The listing builds one solid part. Answer for the finished solid, in the listing's coordinates (mm). Coordinates: 2 decimals unless noted, no trailing zeros. Loops run counter-clockwise (first coordinate to the right, second up) from the corner with the lowest first, then second, coordinate; pieces in that order, holes last. Notation, with made-up numbers: (15.25, 14.5) - (53.25, 14.5) arc R29 ccw to (53.25, 48.5) - close; hole circle Ø7 at (88, 24.25). An arc over 180 degrees is marked (long way). Write each question's results on one line, items separated by ' | '. Start each with the question number.
(1) Find section C-C on z = 14.25. Determine the outline of the cut face in (x, y).
(2) Find section B-B on x = -57.5. Determine the outline of the cut face in (y, z).
(3) Given pin 1 Ø5.5 at (x, y) = (-57.5, 60) entering from +Z; pin 2 Ø12.5 at (x, y) = (57.5, -60) entering from -Z; pin 3 Ø5.5 at (x, y) = (-58.5, -59) entering from +Z, each flat-ended and moving along its own axis, determine where each tip first touches the part or whether it passes through.
(4) Consider line 1 (Y direction, x = 57.5, z = 13.25); line 2 (Y direction, x = -57.5, z = 5.75); line 3 (X direction, y = -62.5, z = 7). Determine where each line is inside the solid, lowest interval first. Write a range as from..to.
(5) Find section A-A on y = -60. Determine the outline of the cut face in (x, z).
from build123d import *

# Parameters (mm, degrees)
SKETCH1_W                                           = 130
SKETCH1_H                                           = 150
EXTRUDE1_DEPTH                                      = 16
CBORE_FOR_M6_HEX_SOCKET_HEAD_CAP_SCREW1_D           = 6.6
CBORE_FOR_M6_HEX_SOCKET_HEAD_CAP_SCREW1_CBORE_D     = 11
CBORE_FOR_M6_HEX_SOCKET_HEAD_CAP_SCREW1_CBORE_DEPTH = 6.4


with BuildPart() as part:
    # Sketch1 → Extrude1 (new body)
    with BuildSketch(Plane.XY):
        Rectangle(SKETCH1_W, SKETCH1_H)
    extrude(amount=EXTRUDE1_DEPTH)

    # CBORE for M6 Hex Socket Head Cap Screw1 (through all)
    with Locations(Plane.XY.offset(16)):
        with Locations((-57.5, 60), (-57.5, 0), (-57.5, -60), (57.5, -60), (57.5, 0), (57.5, 60)):
            CounterBoreHole(CBORE_FOR_M6_HEX_SOCKET_HEAD_CAP_SCREW1_D / 2, CBORE_FOR_M6_HEX_SOCKET_HEAD_CAP_SCREW1_CBORE_D / 2, CBORE_FOR_M6_HEX_SOCKET_HEAD_CAP_SCREW1_CBORE_DEPTH)


solid = part.part
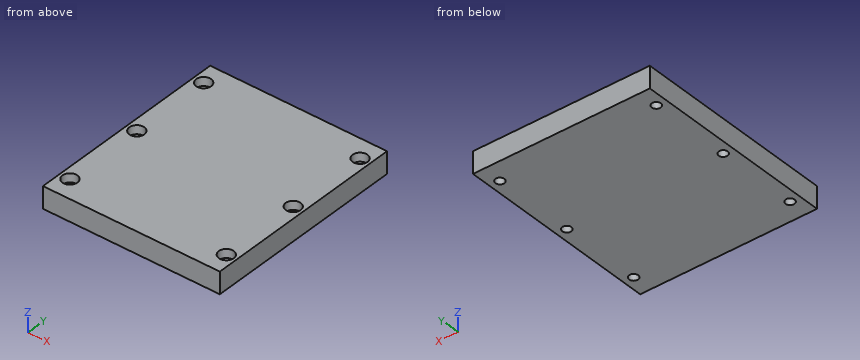
Values:
1) outline: (-65, -75) - (65, -75) - (65, 75) - (-65, 75) - close; hole circle Ø11 at (-57.5, -60); hole circle Ø11 at (-57.5, 0); hole circle Ø11 at (-57.5, 60); hole circle Ø11 at (57.5, -60); hole circle Ø11 at (57.5, 0); hole circle Ø11 at (57.5, 60)
2) outline: (-75, 0) - (-63.3, 0) - (-63.3, 9.6) - (-65.5, 9.6) - (-65.5, 16) - (-75, 16) - close; (-56.7, 0) - (-3.3, 0) - (-3.3, 9.6) - (-5.5, 9.6) - (-5.5, 16) - (-54.5, 16) - (-54.5, 9.6) - (-56.7, 9.6) - close; (3.3, 0) - (56.7, 0) - (56.7, 9.6) - (54.5, 9.6) - (54.5, 16) - (5.5, 16) - (5.5, 9.6) - (3.3, 9.6) - close; (63.3, 0) - (75, 0) - (75, 16) - (65.5, 16) - (65.5, 9.6) - (63.3, 9.6) - close
3) pin 1: passes through | pin 2: stops at z = 0 | pin 3: stops at z = 9.6
4) line 1: y = -75..-65.5, -54.5..-5.5, 5.5..54.5, 65.5..75 | line 2: y = -75..-63.3, -56.7..-3.3, 3.3..56.7, 63.3..75 | line 3: x = -65..-59.65, -55.35..55.35, 59.65..65
5) outline: (-65, 0) - (-60.8, 0) - (-60.8, 9.6) - (-63, 9.6) - (-63, 16) - (-65, 16) - close; (-54.2, 0) - (54.2, 0) - (54.2, 9.6) - (52, 9.6) - (52, 16) - (-52, 16) - (-52, 9.6) - (-54.2, 9.6) - close; (60.8, 0) - (65, 0) - (65, 16) - (63, 16) - (63, 9.6) - (60.8, 9.6) - close
